from build123d import *

# Parameters (mm, degrees)
BOSS_EXTRUDE1_DEPTH = 25.4
SKETCH2_W           = 25.4
SKETCH2_H           = 25.4
SKETCH2_R           = 2.38125
BOSS_EXTRUDE2_DEPTH = 2.54
SKETCH3_R           = 3.175
CUT_EXTRUDE1_DEPTH  = 41.148


with BuildPart() as part:
    # Sketch1 → Boss-Extrude1 (new body)
    with BuildSketch(Plane.XY):
        Polygon((0, 0), (3.175, 0), (3.673626559, -14.278796441), (0.498626559, -14.278796441), align=None)
    extrude(amount=BOSS_EXTRUDE1_DEPTH)

    # Sketch2 → Boss-Extrude2 (add)
    with BuildSketch(Plane(origin=(0, 0, 0), x_dir=(1, 0, 0), z_dir=(0, 1, 0))):
        with Locations((12.7, -12.7)):
            Rectangle(SKETCH2_W, SKETCH2_H)
        with Locations(Location((12.7, -12.7, 0), (0, 0, 270))):
            Circle(SKETCH2_R, mode=Mode.SUBTRACT)
    extrude(amount=BOSS_EXTRUDE2_DEPTH)

    # Sketch3 → Cut-Extrude1 (cut)
    with BuildSketch(Plane(origin=(25.4, 0, 0), x_dir=(0, 0, -1), z_dir=(1, 0, 0))):
        with Locations(Location((-12.7, -7.166796441, 0), (0, 0, 270))):
            Circle(SKETCH3_R)
    extrude(amount=-CUT_EXTRUDE1_DEPTH, mode=Mode.SUBTRACT)


solid = part.part
Source: CAD feature listing. Evaluate the final solid. Frame: model axes, mm. Give positions to 0.01 mm unless a question says otherwise; leave off trailing zeros. Write each loop counter-clockwise with the first axis right and the second up, starting at its lowest first coordinate (ties: lowest second). Pieces come first, ordered by that corner, then holes. Notation, with made-up numbers: M 15.25,-27 L 61.25,-27 A18 ccw 61.25,8 Z; hole C 63,88 d4. An arc over 180 degrees is marked long. Return JSON: item names as keys, results as strings. Group by question number.
1) Material intervals for line 1 along X through (y, z) = (1.25, 12.5); line 2 along Y through (x, z) = (1, 12.7); line 3 along Y through (x, z) = (11, 4.5), sorted ascending. Write a range as [from, to].
2) Cut plane B-B, the plane x = 12.7. Output: boundary loops of the cut face in (y, z), plus the area to 3 significant figures.
3) Cut plane C-C, the plane y = -10. Output: boundary loops of the cut face in (x, z), plus the area to 3 significant figures.
4) Cut plane A-A, the plane z = 20.5. Output: boundary loops of the cut face in (x, y) (3 decimals), plus the area to 3 significant figures.
5) Pull-direction query (Y, two-part tool) for faces 1 (the face through (2, -14.279, 13)), 2 (the face through (7.9, 0.3, 25.4)), 3 (the face through (1.86, -10.1, 13.92)); classes: pulls with the +Y half, pulls with the -Y half, needs draft (parallel to the pull), parting line crosses it, or undercut.
6) Pin query (flat end, axial travel): P1, Ø5.5, axis at x = 12.7, z = 12.7, coming from the -Y side; P2, Ø8, axis at y = -5.5, z = 7, coming from the +X side; P3, Ø8.5, axis at y = -7.17, z = 12.7, coming from the +X side. Return the tip coordinate at first contact, or that it passes through.
7) Cut plane D-D, the plane z = 12.7. Output: boundary loops of the cut face in (x, y) (3 decimals), plus the area to 3 significant figures.
Recorded:
{
 "1": {"line 1": "x = [0, 10.33], [15.07, 25.4]", "line 2": "y = [-14.28, -10.34], [-3.99, 2.54]", "line 3": "y = [0, 2.54]"},
 "2": {"outline": "M 0,0 L 2.54,0 L 2.54,10.32 L 0,10.32 Z; M 0,15.08 L 2.54,15.08 L 2.54,25.4 L 0,25.4 Z", "area": "52.4 mm²"},
 "3": {"outline": "M 0.35,0 L 3.52,0 L 3.52,11.27 L 0.35,11.27 Z; M 0.35,14.13 L 3.52,14.13 L 3.52,25.4 L 0.35,25.4 Z", "area": "71.5 mm²"},
 "4": {"outline": "M 0,0 L 0.499,-14.279 L 3.674,-14.279 L 3.175,0 L 25.4,0 L 25.4,2.54 L 0,2.54 Z", "area": "110 mm²"},
 "5": {"face 1": "pulls with the -Y half", "face 2": "needs draft", "face 3": "undercut"},
 "6": {"P1": "stops at y = 0", "P2": "stops at x = 3.51", "P3": "stops at x = 3.57"},
 "7": {"outline": "M 0,0 L 0.139,-3.992 L 3.314,-3.992 L 3.175,0 L 10.319,0 L 10.319,2.54 L 0,2.54 Z; M 0.361,-10.342 L 0.499,-14.279 L 3.674,-14.279 L 3.536,-10.342 Z; M 15.081,0 L 25.4,0 L 25.4,2.54 L 15.081,2.54 Z", "area": "77.6 mm²"}
}
